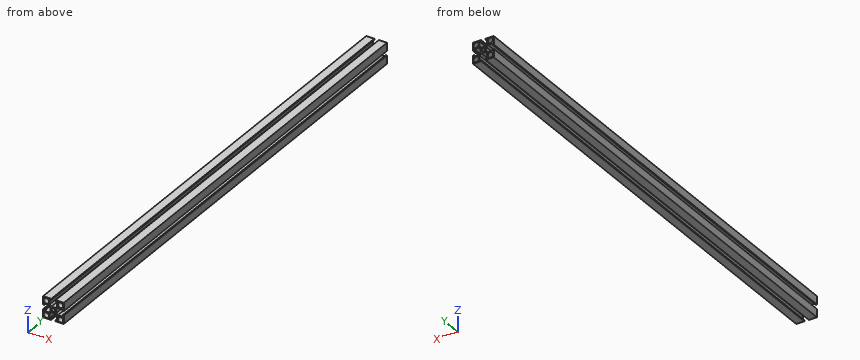
```python
from build123d import *

# Parameters (mm, degrees)
SKETCH_2_R      = 3.8
SKETCH_2_W      = 8.2
SKETCH_2_H      = 8.2
SKETCH_2_R_2    = 2.4
EXTRUDE_1_DEPTH = 740


with BuildPart() as part:
    # 草图2 → 凸台-拉伸1 (new body)
    # profile 1 of 5: a face of its own
    with BuildSketch(Plane(origin=(0, 0, 0), x_dir=(1, 0, 0), z_dir=(0, 1, 0))):
        Polygon((-13.2, -3.15), (-15, -3.15), (-15, -15), (-3.15, -15), (-3.15, -13.2), (-5.25, -13.2), (-5.25, -6.522792206), (-2.827207794, -4.1), (-4.1, -4.1), (-4.1, -2.827207794), (-6.522792206, -5.25), (-13.2, -5.25), align=None)
        with Locations(Location((-10.223905857, -10.223905857, 0), (0, 0, 270))):
            Circle(SKETCH_2_R, mode=Mode.SUBTRACT)
    # profile 2 of 5: a face of its own
    with BuildSketch(Plane(origin=(0, 0, 0), x_dir=(1, 0, 0), z_dir=(0, 1, 0))):
        Rectangle(SKETCH_2_W, SKETCH_2_H)
        with Locations(Location((0, 0, 0), (0, 0, 270))):
            Circle(SKETCH_2_R_2, mode=Mode.SUBTRACT)
    # profile 3 of 5: a face of its own
    with BuildSketch(Plane(origin=(0, 0, 0), x_dir=(1, 0, 0), z_dir=(0, 1, 0))):
        Polygon((15, -15), (15, -3.15), (13.2, -3.15), (13.2, -5.25), (6.522792206, -5.25), (4.1, -2.827207794), (4.1, -4.1), (2.827207794, -4.1), (5.25, -6.522792206), (5.25, -13.2), (3.15, -13.2), (3.15, -15), align=None)
        with Locations(Location((10.223905857, -10.223905857, 0), (0, 0, 270))):
            Circle(SKETCH_2_R, mode=Mode.SUBTRACT)
    # profile 4 of 5: a face of its own
    with BuildSketch(Plane(origin=(0, 0, 0), x_dir=(1, 0, 0), z_dir=(0, 1, 0))):
        Polygon((15, 15), (3.15, 15), (3.15, 13.2), (5.25, 13.2), (5.25, 6.522792206), (2.827207794, 4.1), (4.1, 4.1), (4.1, 2.827207794), (6.522792206, 5.25), (13.2, 5.25), (13.2, 3.15), (15, 3.15), align=None)
        with Locations(Location((10.223905857, 10.223905857, 0), (0, 0, 270))):
            Circle(SKETCH_2_R, mode=Mode.SUBTRACT)
    # profile 5 of 5: a face of its own
    with BuildSketch(Plane(origin=(0, 0, 0), x_dir=(1, 0, 0), z_dir=(0, 1, 0))):
        Polygon((-3.15, 13.2), (-3.15, 15), (-15, 15), (-15, 3.15), (-13.2, 3.15), (-13.2, 5.25), (-6.522792206, 5.25), (-4.1, 2.827207794), (-4.1, 4.1), (-2.827207794, 4.1), (-5.25, 6.522792206), (-5.25, 13.2), align=None)
        with Locations(Location((-10.223905857, 10.223905857, 0), (0, 0, 270))):
            Circle(SKETCH_2_R, mode=Mode.SUBTRACT)
    extrude(amount=EXTRUDE_1_DEPTH)


solid = part.part
```
Here's how the part is built. I have some questions about the finished solid (model axes, mm). Round coordinates to 2 decimals unless told otherwise and drop trailing zeros. Answer as CSV lines item,"result".
1. For pin 1 (3 mm diameter, centred on x = 0.5, y = 345, fed in from +Z), with a flat end and sliding along its axis, tell me the tip position at first contact or that it passes through.
Final values:
pin 1,"stops at z = 4.1"
2. If I drill on L1, parallel to X at y = 165, z = 11.25; L2, parallel to Z at x = 10.75, y = 80, over which ranges is the centre line in solid material (lowest first)?
Final values:
L1,"x = -15 to -13.88, -6.57 to -5.25, 5.25 to 6.57, 13.88 to 15"
L2,"z = -15 to -13.99, -6.46 to -5.25, 5.25 to 6.46, 13.99 to 15"
3. If we section it at A-A on y = 567: Count the separate pieces of the cut face and the enclosed holes in it, plus the area to 3 significant figures.
Final values:
separate pieces,"1"
enclosed holes,"5"
area,"296 mm^2"
